The model under review builds one solid part; all positions refer to its coordinate system, in mm. A direction names the side the tool comes from. Coordinates: 2 decimals unless noted, no trailing zeros. Loops run counter-clockwise (first coordinate to the right, second up) from the corner with the lowest first, then second, coordinate; pieces in that order, holes last. Notation, with made-up numbers: (51.5, 45) - (64.5, 45) arc R11 cw to (64.5, 52) - close; hole circle Ø4 at (27.5, -8). An arc over 180 degrees is marked (long way). One line per item, written item: value. Start each with the question number.
1. Insertion check: P1, Ø0.6, axis at y = -45, z = 1, coming from the +X side; P2, Ø1.2, axis at y = -78, z = 1, coming from the -X side; P3, Ø2, axis at x = 65, y = -21.5, coming from the -Z side; P4, Ø1, axis at x = 52.5, z = 3, coming from the +Y side. Each pin has a flat end and moves straight along its axis. Give the tip position at first contact, or say it passes through.
2. Mouldability with a two-part tool opening along Y and no side actions: class faces 1 (the face through (54, -75, 4)), 2 (the face through (0, -73, 2)), 3 (the face through (54, -90, 2)) as +Y half, -Y half, draft (parallel to the pull), parting line (faces both ways), or undercut.
3. We need section A-A, the plane x = 53. Give the boundary of the cut face in (y, z), then the cut area to 3 significant figures.
4. For faces 4 (the face through (110, -73, 2)), 5 (the face through (54, -30, 2)), 6 (the face through (72, -82, 2)), list the 3-axis set-ups (+Z, -Z, +X, -X, +Y, -Y) from which the entire face can be reached by the end or side of a thin tool; tool diameter is ignored.
5. To check wall thickness, follow line 1 (X direction, y = -77.5, z = 3.7); line 2 (Y direction, x = 54, z = 2.65); line 3 (Y direction, x = 39.5, z = 3.6). State the ranges of each line that lie inside material, in increasing order.
from build123d import *

# Parameters (mm, degrees)
SKETCH_W               = 110
SKETCH_H               = 90
PAD_DEPTH              = 2
PAD001_DEPTH           = 2
PAD002_DEPTH           = 2
LINEARPATTERN_COUNT    = 14
LINEARPATTERN_PITCH    = 6.409401
PAD003_DEPTH           = 2
LINEARPATTERN001_COUNT = 14
LINEARPATTERN001_PITCH = 6.409401


with BuildPart() as part:
    # Sketch → Pad (new body)
    with BuildSketch(Plane.XY):
        with Locations((55, -45)):
            Rectangle(SKETCH_W, SKETCH_H)
    extrude(amount=PAD_DEPTH)

    # Sketch001 (on Face6 of Pad) → Pad001 (join)
    with BuildSketch(Plane.XY.offset(2)):
        Polygon((110, -90), (110, -60), (0, -60), (0, -90), (30, -90), (30, -75), (45, -75), (45, -90), (65, -90), (65, -75), (80, -75), (80, -90), align=None)
    extrude(amount=PAD001_DEPTH)

    # Sketch002 (on Face2 of Pad001) → Pad002 (join)
    with BuildSketch(Plane(origin=(0, 0, 0), x_dir=(0, -1, 0), z_dir=(-1, 0, 0))):
        Polygon((2, 0), (3.154701, 2), (5.154701, 2), (6.309401, 0), align=None)
    pad002 = extrude(amount=PAD002_DEPTH)

    # LinearPattern: Pad002 ×14
    with Locations(*[(0, -i * LINEARPATTERN_PITCH, 0) for i in range(1, LINEARPATTERN_COUNT)]):
        add(pad002)

    # Sketch003 (on Face3 of LinearPattern) → Pad003 (join)
    with BuildSketch(Plane.YZ.offset(110)):
        Polygon((-2, 0), (-3.154701, 2), (-5.154701, 2), (-6.309401, 0), align=None)
    pad003 = extrude(amount=PAD003_DEPTH)

    # LinearPattern001: Pad003 ×14
    with Locations(*[(0, -i * LINEARPATTERN001_PITCH, 0) for i in range(1, LINEARPATTERN001_COUNT)]):
        add(pad003)


solid = part.part
Findings below:
1. P1: x = 110
1. P2: x = 0
1. P3: z = 0
1. P4: y = -60
2. face 1: draft
2. face 2: undercut
2. face 3: -Y half
3. outline: (-90, 0) - (0, 0) - (0, 2) - (-60, 2) - (-60, 4) - (-90, 4) - close
3. area: 240 mm2
4. face 4: +Z, +X
4. face 5: +Z, +X, -X, +Y
4. face 6: +Z, -Y
5. line 1: 0 to 30, 45 to 65, 80 to 110
5. line 2: -90 to -60
5. line 3: -75 to -60
